Print and shaded views of the part. All mm, measured from the part's lowest x, y and z. A direction names the side the tool comes from. Round coordinates to 2 decimals unless told otherwise and drop trailing zeros. Loops run counter-clockwise (first coordinate to the right, second up) from the corner with the lowest first, then second, coordinate; pieces in that order, holes last. Notation, with made-up numbers: (49, 59.5) - (65, 59.5) arc R18 ccw to (65, 94.5) - close; hole circle Ø11 at (-7, 52). An arc over 180 degrees is marked (long way). Put each result on its own line as item: value. Start each with the question number.
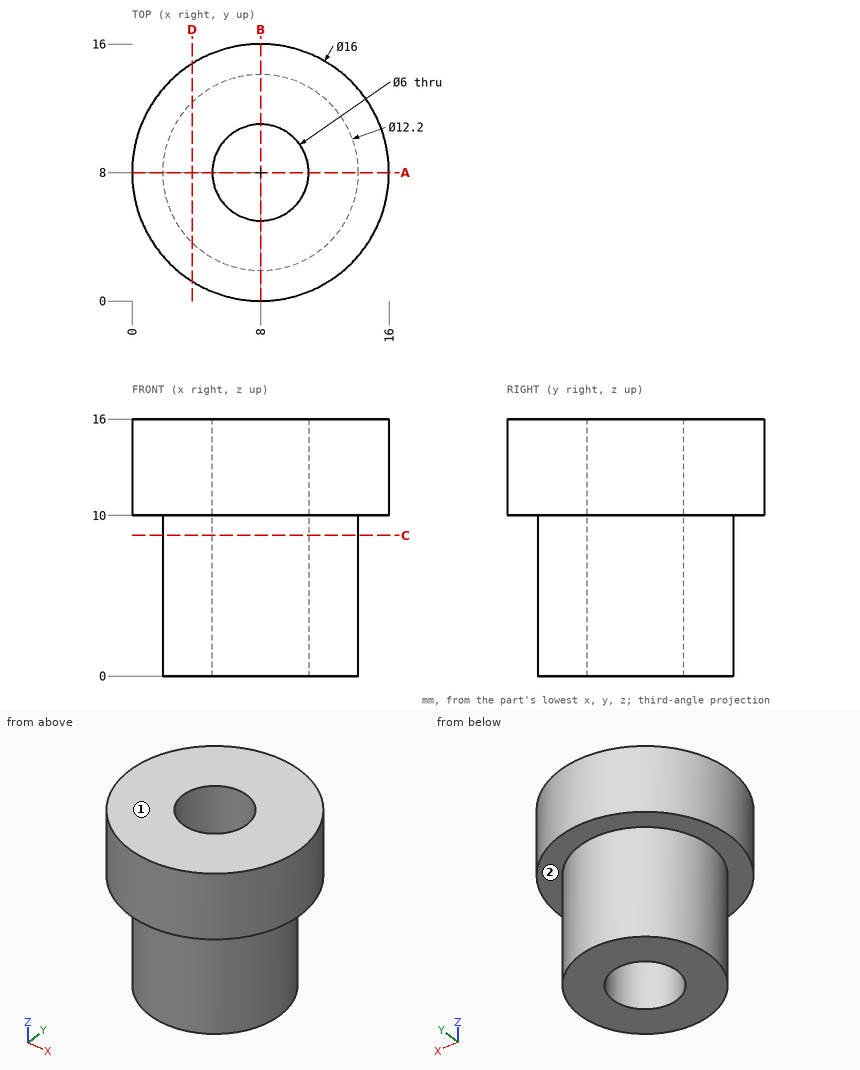
Item 1: Slice it at D-D (x = 3.75). Give the cut face in (y, z), plus the area to 3 significant figures.
Item 2: Slice it at C-C (z = 8.75). Give the cut face in (x, y).
Item 3: Drop flat-ended pins along their axis: pin 1 Ø5.5 at (x, y) = (8, 8) entering from -Z; pin 2 Ø8 at (x, z) = (6.5, 9.5) entering from +Y; pin 3 Ø1 at (x, y) = (3.5, 14) entering from -Z; pin 4 Ø2 at (y, z) = (6, 9.5) entering from +X. Give the stop position or say it passes through.
Item 4: Slice it at A-A (y = 8). Give the cut face in (x, z), plus the area to 3 significant figures.
Item 5: Drill centre lines: probe 1 along Y at (x, z) = (8, 10.25); probe 2 along Y at (x, z) = (8, 3.5); probe 3 along Z at (x, y) = (3.25, 12.5). Where is each one in solid material? Low to high. Write a range as [from, to].
Item 6: Which spindle directions (+Z, -Z, +X, -X, +Y, -Y) get a long thin tool onto all of the face, cutting with end or side? Do the marked faces 1 and 2. Say none if no direction does.
Computed values:
1. outline: (1.22, 10) - (3.62, 10) - (3.62, 0) - (12.38, 0) - (12.38, 10) - (14.78, 10) - (14.78, 16) - (1.22, 16) - close
1. area: 169 mm^2
2. outline: circle Ø12.2 at (8, 8); hole circle Ø6 at (8, 8)
3. pin 1: passes through
3. pin 2: stops at y = 16
3. pin 3: stops at z = 10
3. pin 4: stops at x = 15.92
4. outline: (0, 10) - (1.9, 10) - (1.9, 0) - (5, 0) - (5, 16) - (0, 16) - close; (11, 0) - (14.1, 0) - (14.1, 10) - (16, 10) - (16, 16) - (11, 16) - close
4. area: 122 mm^2
5. probe 1: y = [0, 5], [11, 16]
5. probe 2: y = [1.9, 5], [11, 14.1]
5. probe 3: z = [10, 16]
6. face 1: +Z, +X, -X, +Y, -Y
6. face 2: -Z
